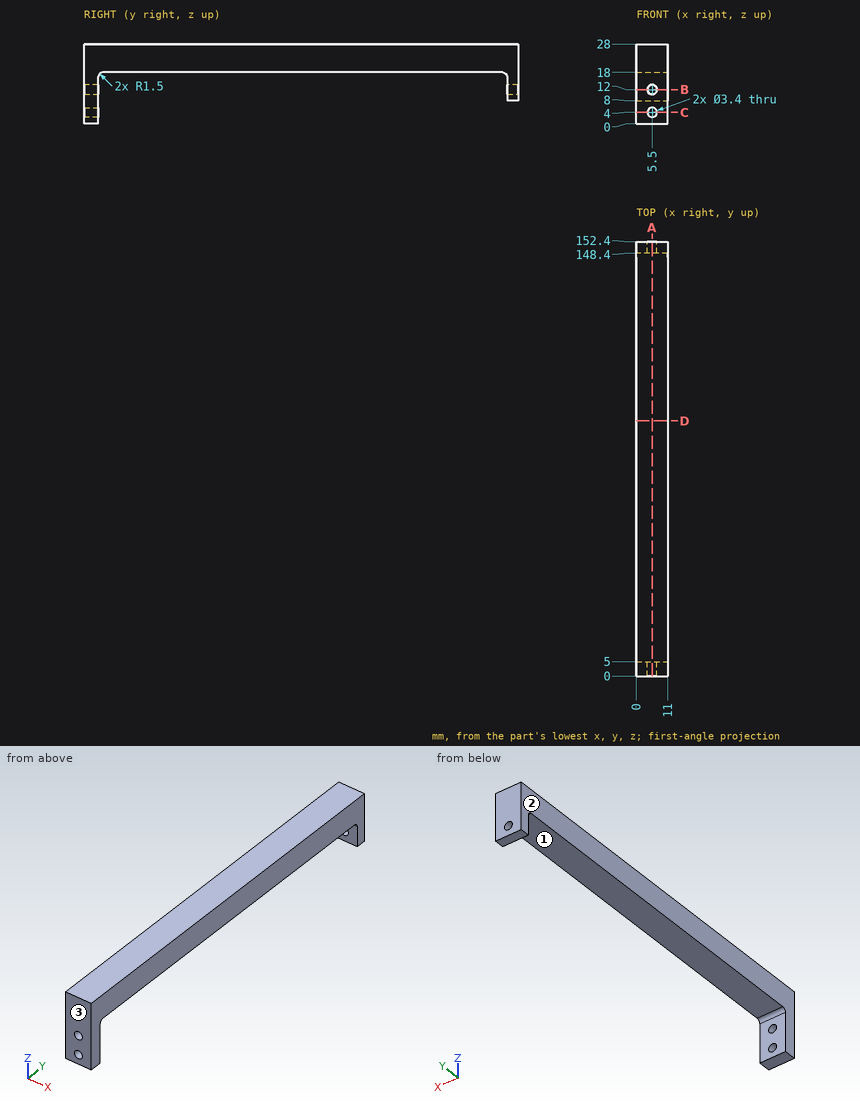
Geometry check sheet. Reference: drawing and pictorial views, mm from the part's lowest x, y, z. Give positions to 0.01 mm unless a question says otherwise; leave off trailing zeros. Order: outer loops, then holes, each group sorted by start corner. A loop starts at its lowest first (then second) coordinate and runs counter-clockwise, first axis right, second up. Notation, with made-up numbers: M 22.25,82 L 53.25,82 A24 cw 53.25,108 Z; hole C 18.5,32.5 d10. An arc over 180 degrees is marked long. Answer as a JSON object with one key per item and string values. Group by question number.
1) Mould release check, pull along Y, two halves, no side actions. Record for the marked faces 1, 2 and 3: released by +Y, released by -Y, zero draft, split by the parting line, or undercut.
2) Cross-section at B-B (z = 12). Enter the section's corners in (x, y).
3) Scan lines: line 1 along X through (y, z) = (149.5, 12); line 2 along Y through (x, z) = (1, 11.5); line 3 along Z through (x, y) = (1, 46). Record each from-to range of solid material in increasing order. Write a range as [from, to].
4) Cross-section at A-A (x = 5.5). Enter the section's corners in (y, z), then the cut area to 3 significant figures.
5) Cross-section at D-D (y = 89.5). Enter the section's corners in (x, z).
6) Depth check by flat-ended pin: pin 1 Ø6 at (x, y) = (6.5, 25) entering from -Z; pin 2 Ø2.5 at (x, z) = (5.5, 12) entering from +Y; pin 3 Ø5.5 at (x, z) = (6.5, 5) entering from +Y; pin 4 Ø1.2 at (x, y) = (5.5, 149.5) entering from -Z. Enter the tip coordinate at first touch or a pass-through.
7) Cross-section at C-C (z = 4). Enter the section's corners in (x, y), then the cut area to 3 significant figures.
Result sheet:
{
 "1": {"face 1": "undercut", "face 2": "zero draft", "face 3": "released by -Y"},
 "2": {"outline": "M 0,0 L 3.8,0 L 3.8,5 L 0,5 Z; M 0,148.4 L 3.8,148.4 L 3.8,152.4 L 0,152.4 Z; M 7.2,0 L 11,0 L 11,5 L 7.2,5 Z; M 7.2,148.4 L 11,148.4 L 11,152.4 L 7.2,152.4 Z"},
 "3": {"line 1": "x = [0, 3.8], [7.2, 11]", "line 2": "y = [0, 5], [148.4, 152.4]", "line 3": "z = [18, 28]"},
 "4": {"outline": "M 0,0 L 5,0 L 5,2.3 L 0,2.3 Z; M 0,5.7 L 5,5.7 L 5,10.3 L 0,10.3 Z; M 0,13.7 L 5,13.7 L 5,16.5 A1.5 cw 6.5,18 L 146.9,18 A1.5 cw 148.4,16.5 L 148.4,13.7 L 152.4,13.7 L 152.4,28 L 0,28 Z; M 148.4,8 L 152.4,8 L 152.4,10.3 L 148.4,10.3 Z", "area": "1,610 mm2"},
 "5": {"outline": "M 0,18 L 11,18 L 11,28 L 0,28 Z"},
 "6": {"pin 1": "stops at z = 18", "pin 2": "passes through", "pin 3": "stops at y = 5", "pin 4": "stops at z = 8"},
 "7": {"outline": "M 0,0 L 3.8,0 L 3.8,5 L 0,5 Z; M 7.2,0 L 11,0 L 11,5 L 7.2,5 Z", "area": "38.0 mm2"}
}
